Geometry check sheet. Reference: the model listing, model coordinates, mm. A direction names the side the tool comes from. Round coordinates to 2 decimals unless told otherwise and drop trailing zeros. Write each loop counter-clockwise with the first axis right and the second up, starting at its lowest first coordinate (ties: lowest second). Pieces come first, ordered by that corner, then holes.
from build123d import *

# Parameters (mm, degrees)
SKETCH2_W           = 1
SKETCH2_H           = 3
CUT_EXTRUDE1_DEPTH  = 1
SKETCH3_R           = 0.6
BOSS_EXTRUDE1_DEPTH = 11
CUT_EXTRUDE2_START  = 1.15
SKETCH4_R           = 0.6
SKETCH4_R_2         = 0.5
CUT_EXTRUDE2_DEPTH  = 11.052678251
CHAMFER1_SIZE       = 0.2


with BuildPart() as part:
    # Sketch1 → Revolve1 (revolve)
    with BuildSketch(Plane(origin=(0, 0, 0), x_dir=(1, 0, 0), z_dir=(0, 1, 0))):
        Polygon((0, 0), (-1.5, 0), (-1.5, 1.77), (-0.75, 1.77), (-0.75, 4.37), (-0.5, 4.37), (-0.5, 4.52), (-0.75, 4.52), (-0.75, 4.72), (0, 4.72), align=None)
    revolve(axis=Axis((0, 0, -4.72), (0, 0, 1)))

    # Sketch2 → Cut-Extrude1 (cut)
    with BuildSketch(Plane.XY):
        with Locations((-1.5, 0)):
            Rectangle(SKETCH2_W, SKETCH2_H)
        with Locations((1.5, 0)):
            Rectangle(SKETCH2_W, SKETCH2_H)
    extrude(amount=-CUT_EXTRUDE1_DEPTH, mode=Mode.SUBTRACT)

    # Sketch3 → Boss-Extrude1 (add)
    with BuildSketch(Plane.XY):
        Circle(SKETCH3_R)
    extrude(amount=BOSS_EXTRUDE1_DEPTH)

    # Sketch4 → Cut-Extrude2 (cut, through all)
    with BuildSketch(Plane.XY.offset(CUT_EXTRUDE2_START)):
        Circle(SKETCH4_R)
        with Locations(Location((0, 0, 0), (0, 0, 180))):
            Circle(SKETCH4_R_2, mode=Mode.SUBTRACT)
    extrude(amount=CUT_EXTRUDE2_DEPTH, mode=Mode.SUBTRACT)

    # Chamfer1
    chamfer1_edges = [part.edges().sort_by_distance(p)[0] for p in [
        (0.5, 0, 11),
    ]]
    chamfer(chamfer1_edges, length=CHAMFER1_SIZE)


solid = part.part
1. Depth check by flat-ended pin: pin 1 Ø1 at (x, y) = (0.5, 0) entering from +Z; pin 2 Ø0.6 at (x, y) = (-1, 0) entering from +Z. Enter the tip coordinate at first touch or a pass-through.
2. Section check A-A (y = 0.9). Record the cut outline in (x, z), plus the area to 3 significant figures.
3. Section check C-C (z = 8). Record the cut outline in (x, y).
4. Section check B-B (x = 0). Record the cut outline in (y, z), plus the area to 4 significant figures.
5. Access from +Z, -Z, +X, -X, +Y, -Y to the whole of each face (thin tool, end or side, straight path). Record for faces 1 (the face through (0.108, 0.488, 5.907)), 2 (the face through (1, 0, -0.5)), 3 (the face through (-1, 0, -0.5)), 4 (the face through (0.75, -0.03, -3.09)).
6. Scan lines: line 1 along Z through (x, y) = (0.85, -0.45); line 2 along Z through (x, y) = (1.3, 0.2); line 3 along X through (y, z) = (-1.3, -1.5). Record each from-to range of solid material in increasing order.
Results below:
1. pin 1: stops at z = 11
1. pin 2: stops at z = 0
2. outline: (-1.2, -1.77) - (1.2, -1.77) - (1.2, -1) - (1, -1) - (1, 0) - (-1, 0) - (-1, -1) - (-1.2, -1) - close
2. area: 3.85 mm2
3. outline: circle Ø1 at (0, 0)
4. outline: (-1.5, -1.77) - (-0.75, -1.77) - (-0.75, -4.37) - (-0.5, -4.37) - (-0.5, -4.52) - (-0.75, -4.52) - (-0.75, -4.72) - (0.75, -4.72) - (0.75, -4.52) - (0.5, -4.52) - (0.5, -4.37) - (0.75, -4.37) - (0.75, -1.77) - (1.5, -1.77) - (1.5, 0) - (0.6, 0) - (0.6, 1.15) - (0.5, 1.15) - (0.5, 10.8) - (0.3, 11) - (-0.3, 11) - (-0.5, 10.8) - (-0.5, 1.15) - (-0.6, 1.15) - (-0.6, 0) - (-1.5, 0) - close
4. area: 20.85 mm2
5. face 1: +Z
5. face 2: +Z, +X, +Y, -Y
5. face 3: +Z, -X, +Y, -Y
5. face 4: -Z
6. line 1: z = -1.77 to 0
6. line 2: z = -1.77 to -1
6. line 3: x = -0.75 to 0.75
